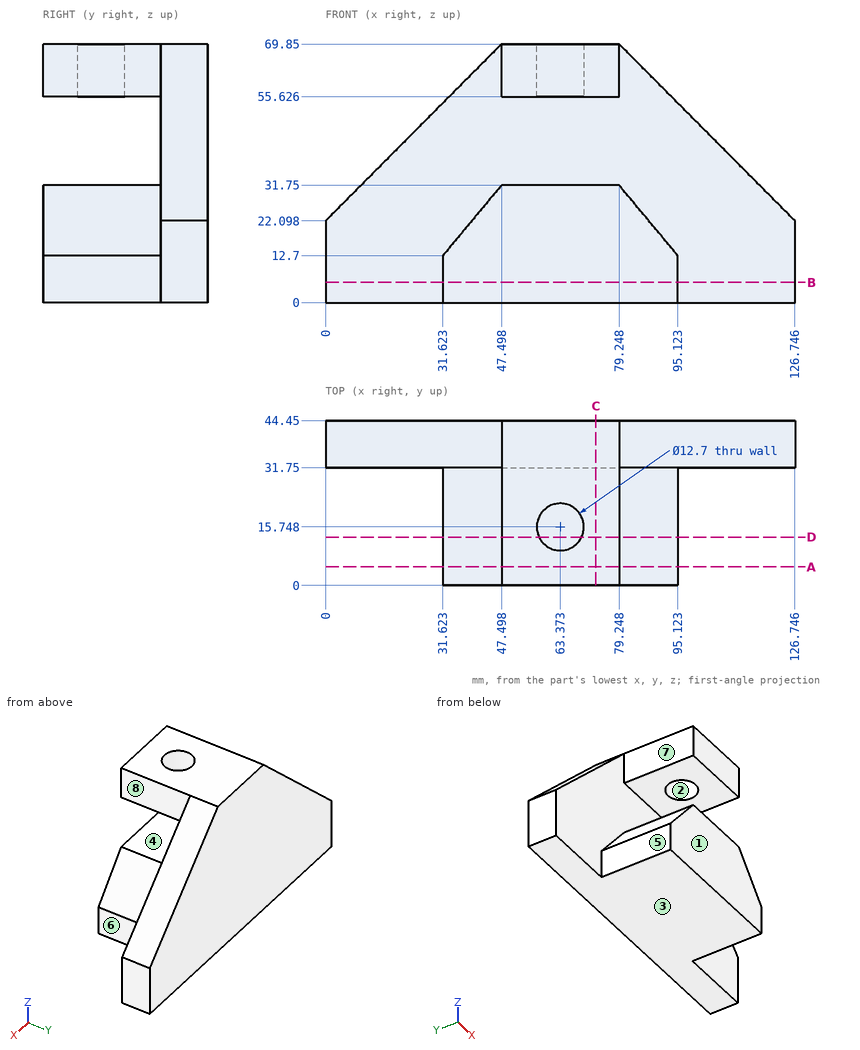
Drawing for the job (mm, zero at the part's lowest x, y, z). A direction names the side the tool comes from. Round coordinates to 2 decimals unless told otherwise and drop trailing zeros. Loops run counter-clockwise (first coordinate to the right, second up) from the corner with the lowest first, then second, coordinate; pieces in that order, holes last.
1. Wall check: probe 1 along X at (y, z) = (28, 60.5); probe 2 along Y at (x, z) = (85.5, 34); probe 3 along Z at (x, y) = (76.5, 15). Give the ranges that are in metal, low to high.
Check values:
probe 1: x = 47.5 to 79.25
probe 2: y = 31.75 to 44.45
probe 3: z = 0 to 31.75, 55.63 to 69.85
2. Band-saw the part on A-A, the plane y = 5. List the corners of the cut face in (x, z), and give its area (3 significant figures).
Check values:
outline: (31.62, 0) - (95.12, 0) - (95.12, 12.7) - (79.25, 31.75) - (47.5, 31.75) - (31.62, 12.7) - close; (47.5, 55.63) - (79.25, 55.63) - (79.25, 69.85) - (47.5, 69.85) - close
area: 2,170 mm2
3. Drop flat-ended pins along their axis: P1, Ø11.5, axis at y = 11.5, z = 65, coming from the +X side; P2, Ø10, axis at y = 8.5, z = 8, coming from the +X side; P3, Ø4, axis at y = 19.5, z = 14.5, coming from the -X side. Give the stop position or say it passes through.
Check values:
P1: stops at x = 79.25
P2: stops at x = 95.12
P3: stops at x = 31.62
4. Band-saw the part on B-B, the plane z = 5.5. List the corners of the cut face in (x, y).
Check values:
outline: (0, 31.75) - (31.62, 31.75) - (31.62, 0) - (95.12, 0) - (95.12, 31.75) - (126.75, 31.75) - (126.75, 44.45) - (0, 44.45) - close
5. Band-saw the part on C-C, the plane x = 73. List the corners of the cut face in (y, z).
Check values:
outline: (0, 0) - (44.45, 0) - (44.45, 69.85) - (0, 69.85) - (0, 55.63) - (31.75, 55.63) - (31.75, 31.75) - (0, 31.75) - close
6. Mould opens along Y. For the marked faces 1, 2 and 3 say: +Y half, -Y half, draft (parallel to the pull), parting line (faces both ways), or undercut.
Check values:
face 1: -Y half
face 2: undercut
face 3: draft
7. Tool access for the marked faces 4, 5, 6, 7 and 8: list every direction of +Z, -Z, +X, -X, +Y, -Y with a clear straight run to the whole face (end or side of a thin tool).
Check values:
face 4: +X, -X, -Y
face 5: +Z, -Z, -X, -Y
face 6: +Z, -Z, +X, -Y
face 7: +Z, -X, -Y
face 8: +Z, +X, -Y
8. Band-saw the part on D-D, the plane y = 13. List the corners of the cut face in (x, z), and give its area (3 significant figures).
Check values:
outline: (31.62, 0) - (95.12, 0) - (95.12, 12.7) - (79.25, 31.75) - (47.5, 31.75) - (31.62, 12.7) - close; (47.5, 55.63) - (57.65, 55.63) - (57.65, 69.85) - (47.5, 69.85) - close; (69.1, 55.63) - (79.25, 55.63) - (79.25, 69.85) - (69.1, 69.85) - close
area: 2,000 mm2
